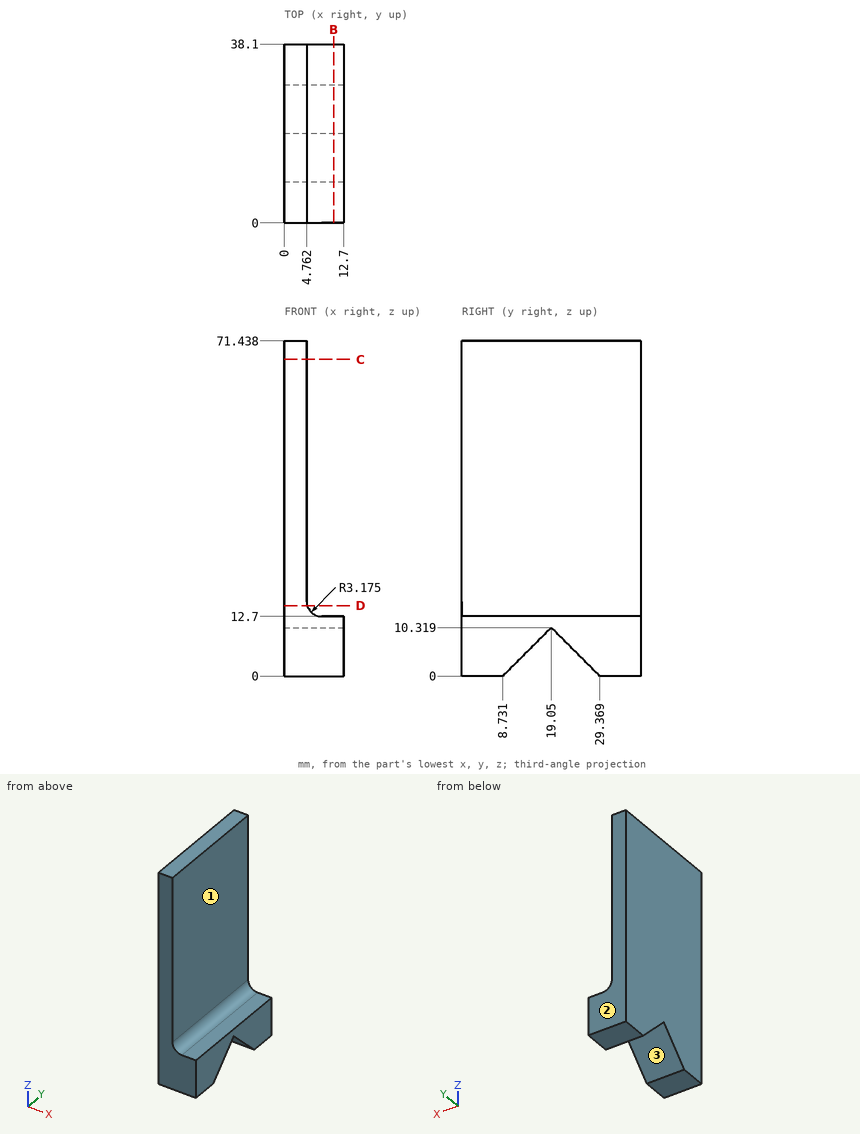
Check sheet for the drawn part. Datum: minimum x, y, z corner. Units: mm. Give positions to 0.01 mm unless a question says otherwise; leave off trailing zeros. Write each loop counter-clockwise with the first axis right and the second up, starting at its lowest first coordinate (ties: lowest second). Pieces come first, ordered by that corner, then holes. Notation, with made-up numbers: (20.5, 2.5) -> (39.5, 2.5) arc R26 cw to (39.5, 21.5) -> close; hole circle Ø7 at (0.5, 25). An arc over 180 degrees is marked (long way). Use one line per item in the form item = value. Start each with the question number.
1. Section check D-D (z = 15). Record the cut outline in (x, y) (1 decimal).
2. Thickness scan on line 1 along X through (y, z) = (15.5, 29); line 2 along Y through (x, z) = (3.5, 6); line 3 along Z through (x, y) = (9.5, 36). Record the ranges inside material, lowest first. Write a range as from..to.
3. Mould release check, pull along Y, two halves, no side actions. Record for the marked faces 1, 2 and 3: pulls with the +Y half, pulls with the -Y half, needs draft (parallel to the pull), parting line crosses it, or undercut.
4. Go/stop test with flat-tipped pins: P1, Ø6, axis at y = 14.5, z = 59.5, coming from the +X side; P2, Ø4, axis at x = 8.5, y = 7, coming from the +Z side (1 decimal); P3, Ø1.4, axis at x = 9.5, y = 25, coming from the +Z side. Record where each tip stops, or that it passes through.
5. Section check C-C (z = 67.5). Record the cut outline in (x, y).
6. Section check B-B (x = 10.5). Record the cut outline in (y, z).
Conclusion:
q1.outline = (0, 0) -> (4.9, 0) -> (4.9, 38.1) -> (0, 38.1) -> close
q2.line_1 = 0..4.76
q2.line_2 = 0..14.73, 23.37..38.1
q2.line_3 = 0..12.7
q3.face_1 = needs draft
q3.face_2 = pulls with the +Y half
q3.face_3 = undercut
q4.P1 = 4.76
q4.P2 = 13
q4.P3 = 12.7
q5.outline = (0, 0) -> (4.76, 0) -> (4.76, 38.1) -> (0, 38.1) -> close
q6.outline = (0, 0) -> (8.73, 0) -> (19.05, 10.32) -> (29.37, 0) -> (38.1, 0) -> (38.1, 12.7) -> (0, 12.7) -> close
